The model under review builds one solid part; all positions refer to its coordinate system, in mm. Face numbers are marked on the shaded views. A direction names the side the tool comes from. Give positions to 0.01 mm unless a question says otherwise; leave off trailing zeros. Loops run counter-clockwise (first coordinate to the right, second up) from the corner with the lowest first, then second, coordinate; pieces in that order, holes last. Notation, with made-up numbers: M -9,-37 L 7,-37 A33 ccw 7,-2 Z; hole C -18.5,11.25 d3. An arc over 180 degrees is marked long. One line per item, written item: value. Start each with the question number.
Q1. To check wall thickness, follow line 1 along Y through (x, z) = (-1, -0.2); line 2 along X through (y, z) = (-1.75, -0.25); line 3 along Z through (x, y) = (4.25, -2.5). State the ranges of each line that lie inside material, in increasing order. Write a range as from..to.
Q2. For pin 1 (1 mm diameter, centred on y = -1.5, z = -1, fed in from -X); pin 2 (1.1 mm diameter, centred on y = -5, z = -1, fed in from -X); pin 3 (0.6 mm diameter, centred on x = 2.5, z = -1.5, fed in from +Y), all flat-tipped, find the tip position at first contact; note any pin that passes through.
Q3. Mouldability with a two-part tool opening along Y and no side actions: class the marked faces 3, 4, 5 and 6 as released by +Y, released by -Y, zero draft, split by the parting line, or undercut.
Q4. We need section B-B on y = 2.75. Write out the cut boundary in (x, z).
Q5. We need section A-A on z = -0.75. Write out the cut boundary in (x, y), plus the area to 3 significant figures.
Q6. We need section C-C on x = -3.5. Write out the cut boundary in (y, z).
Q7. For the marked faces 1 and 2, list the 3-axis set-ups (+Z, -Z, +X, -X, +Y, -Y) from which the entire face can be reached by the end or side of a thin tool; tool diameter is ignored.
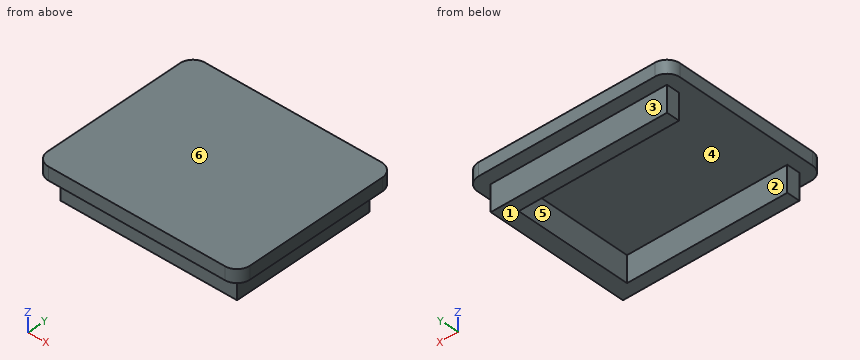
```python
from build123d import *

# Parameters (mm, degrees)
ESQUISSE2_W        = 15.5
ESQUISSE2_H        = 13
BOSS_EXTRU_1_DEPTH = 1
BOSS_EXTRU_2_DEPTH = 2
CONG_1_R           = 1


with BuildPart() as part:
    # Esquisse2 → Boss.-Extru.1 (new body)
    with BuildSketch(Plane.XY):
        Rectangle(ESQUISSE2_W, ESQUISSE2_H)
    extrude(amount=BOSS_EXTRU_1_DEPTH)

    # Esquisse3 → Boss.-Extru.2 (add)
    with BuildSketch(Plane(origin=(0, 0, 0), x_dir=(-1, 0, 0), z_dir=(0, 0, -1))):
        Polygon((5.522727273, -4.5), (6.75, -4.5), (6.75, -5.5), (-6.75, -5.5), (-6.75, 5.5), (6.75, 5.5), (6.75, 4.5), (5.522727273, 4.5), (-5.522727273, 4.5), (-5.522727273, -4.5), align=None)
    extrude(amount=BOSS_EXTRU_2_DEPTH)

    # Congé1
    cong_1_edges = [part.edges().sort_by_distance(p)[0] for p in [
        (-7.75, 6.5, 0.5),
        (7.75, 6.5, 0.5),
        (7.75, -6.5, 0.5),
        (-7.75, -6.5, 0.5),
    ]]
    fillet(cong_1_edges, radius=CONG_1_R)


solid = part.part
```
Solved:
1. line 1: -5.5..-4.5, 4.5..5.5
1. line 2: 5.52..6.75
1. line 3: 0..1
2. pin 1: x = 5.52
2. pin 2: x = -6.75
2. pin 3: y = 5.5
3. face 3: released by +Y
3. face 4: undercut
3. face 5: undercut
3. face 6: zero draft
4. outline: M -7.75,0 L 5.52,0 L 5.52,-2 L 6.75,-2 L 6.75,0 L 7.75,0 L 7.75,1 L -7.75,1 Z
5. outline: M -6.75,-5.5 L 6.75,-5.5 L 6.75,5.5 L -6.75,5.5 L -6.75,4.5 L 5.52,4.5 L 5.52,-4.5 L -6.75,-4.5 Z
5. area: 38.0 mm2
6. outline: M -6.5,0 L -5.5,0 L -5.5,-2 L -4.5,-2 L -4.5,0 L 4.5,0 L 4.5,-2 L 5.5,-2 L 5.5,0 L 6.5,0 L 6.5,1 L -6.5,1 Z
7. face 1: -Z, +X, -X, +Y, -Y
7. face 2: -Z, -X
